from build123d import *

# Parameters (mm, degrees)
F0_W     = 70
F0_H     = 70
F1_DEPTH = 2.5
F2_W     = 5
F2_H     = 10
F3_DEPTH = 5
F4_W     = 10
F4_H     = 5
F5_DEPTH = 5
F7_D     = 3.4


with BuildPart() as f1:
    # F0 (on Top) → F1 (new body, symmetric)
    with BuildSketch(Plane.XY):
        Rectangle(F0_W, F0_H)
    extrude(amount=F1_DEPTH, both=True)

    # F2 (on face) → F3 (join, through all)
    with BuildSketch(Plane(origin=(0, 0, -2.5), x_dir=(1, 0, 0), z_dir=(0, 0, -1))):
        with Locations((-37.5, -30)):
            Rectangle(F2_W, F2_H)
        with Locations((37.5, -30)):
            Rectangle(F2_W, F2_H)
        with Locations((37.5, -10)):
            Rectangle(F2_W, F2_H)
        with Locations((-37.5, -10)):
            Rectangle(F2_W, F2_H)
        with Locations((37.5, 10)):
            Rectangle(F2_W, F2_H)
        with Locations((-37.5, 10)):
            Rectangle(F2_W, F2_H)
        with Locations((37.5, 30)):
            Rectangle(F2_W, F2_H)
        with Locations((-37.5, 30)):
            Rectangle(F2_W, F2_H)
    extrude(amount=-F3_DEPTH)

    # F4 (on face) → F5 (join, through all)
    with BuildSketch(Plane(origin=(0, 0, -2.5), x_dir=(1, 0, 0), z_dir=(0, 0, -1))):
        with Locations((-30, 37.5)):
            Rectangle(F4_W, F4_H)
        with Locations((-10, 37.5)):
            Rectangle(F4_W, F4_H)
        with Locations((10, 37.5)):
            Rectangle(F4_W, F4_H)
        with Locations((30, 37.5)):
            Rectangle(F4_W, F4_H)
    extrude(amount=-F5_DEPTH)

    # F7 (through all)
    with Locations(Plane(origin=(0, 0, -2.5), x_dir=(1, 0, 0), z_dir=(0, 0, -1))):
        with Locations((-26.5, 26.5), (26.5, 26.5), (26.5, -26.5), (-26.5, -26.5)):
            Hole(F7_D / 2)


solid = f1.part
Here's how the part is built. I have some questions about the finished solid (model axes, mm). A direction names the side the tool comes from. Give positions to 0.01 mm unless a question says otherwise; leave off trailing zeros. Loops run counter-clockwise (first coordinate to the right, second up) from the corner with the lowest first, then second, coordinate; pieces in that order, holes last. Notation, with made-up numbers: (80, 89) -> (133, 89) arc R23 cw to (133, 97) -> close; hole circle Ø2 at (72.5, -39). An arc over 180 degrees is marked (long way). Answer as a JSON object with one key per item and string values. Group by question number.
Item 1: Imagine slicing it at D-D on x = -1. Write out the boundary of the cut face in (y, z), then the cut area to 3 significant figures.
Item 2: Imagine slicing it at C-C on z = 1.35. Give the number of separate pieces and of enclosed holes in the cut face, then the cut area to 3 significant figures.
Item 3: Will these pins go through, and if not, where does the flat tip stop? pin 1 (1.5 mm diameter, centred on y = -17.5, z = -1, fed in from +X); pin 2 (1.5 mm diameter, centred on y = -37.5, z = 0.5, fed in from -X); pin 3 (2.5 mm diameter, centred on x = -38.5, z = 0.5, fed in from -Y).
Item 4: I need wall thicknesses on L1, parallel to X at y = -26.5, z = -0.55; L2, parallel to Y at x = 26.5, z = -0.5; L3, parallel to X at y = -27, z = 0.9. Which ranges of each line are inside material? Lowest first, please.
Item 5: Imagine slicing it at B-B on y = -26.5. Write out the boundary of the cut face in (x, z).
Item 6: Thinking about a two-plate mould opening in Y: for faces 5 (the flat face through (20, -35, 0)), 6 (the flat face through (25, -37, 0)), 7 (the cylindrical face through (-27.414, 25.067, 0.035)), which applies, pulls with the +Y half, pulls with the -Y half, needs draft (parallel to the pull), parting line crosses it, or undercut?
Item 7: On a 3-axis mill with a long thin cutter (end or side, diameter ignored), from which of +Z, -Z, +X, -X, +Y, -Y can I reach the whole of each face in a straight line? I mean faces 1 (the flat face through (-25, -37, 0)), 2 (the flat face through (-35, 0, 0)), 3 (the flat face through (35, 0, 0)), 4 (the flat face through (40, -30, 0)). Say none if no direction works.
Item 8: Imagine slicing it at A-A on x = 26.5. Write out the boundary of the cut face in (y, z), then the cut area to 3 significant figures.
Answer list:
{
 "1": {"outline": "(-35, -2.5) -> (35, -2.5) -> (35, 2.5) -> (-35, 2.5) -> close", "area": "350 mm2"},
 "2": {"separate pieces": "1", "enclosed holes": "4", "area": "5,460 mm2"},
 "3": {"pin 1": "stops at x = 35", "pin 2": "stops at x = -35", "pin 3": "stops at y = -35"},
 "4": {"L1": "x = -40 to -28.2, -24.8 to 24.8, 28.2 to 40", "L2": "y = -40 to -28.2, -24.8 to 24.8, 28.2 to 35", "L3": "x = -40 to -28.12, -24.88 to 24.88, 28.12 to 40"},
 "5": {"outline": "(-40, -2.5) -> (-28.2, -2.5) -> (-28.2, 2.5) -> (-40, 2.5) -> close; (-24.8, -2.5) -> (24.8, -2.5) -> (24.8, 2.5) -> (-24.8, 2.5) -> close; (28.2, -2.5) -> (40, -2.5) -> (40, 2.5) -> (28.2, 2.5) -> close"},
 "6": {"face 5": "pulls with the -Y half", "face 6": "needs draft", "face 7": "undercut"},
 "7": {"face 1": "+Z, -Z, -Y", "face 2": "+Z, -Z, -X", "face 3": "+Z, -Z, +X", "face 4": "+Z, -Z, +X, +Y, -Y"},
 "8": {"outline": "(-40, -2.5) -> (-28.2, -2.5) -> (-28.2, 2.5) -> (-40, 2.5) -> close; (-24.8, -2.5) -> (24.8, -2.5) -> (24.8, 2.5) -> (-24.8, 2.5) -> close; (28.2, -2.5) -> (35, -2.5) -> (35, 2.5) -> (28.2, 2.5) -> close", "area": "341 mm2"}
}
